The model under review builds one solid part; all positions refer to its coordinate system, in mm. Face numbers are marked on the shaded views. Give positions to 0.01 mm unless a question says otherwise; leave off trailing zeros. Write each loop counter-clockwise with the first axis right and the second up, starting at its lowest first coordinate (ties: lowest second). Pieces come first, ordered by that corner, then holes. Notation, with made-up numbers: (48.25, 59) - (91.25, 59) arc R30 cw to (91.25, 88) - close; hole circle Ø6 at (34, -25.75). An arc over 180 degrees is marked (long way). One line per question, with ' | ' between items. Start each with the question number.
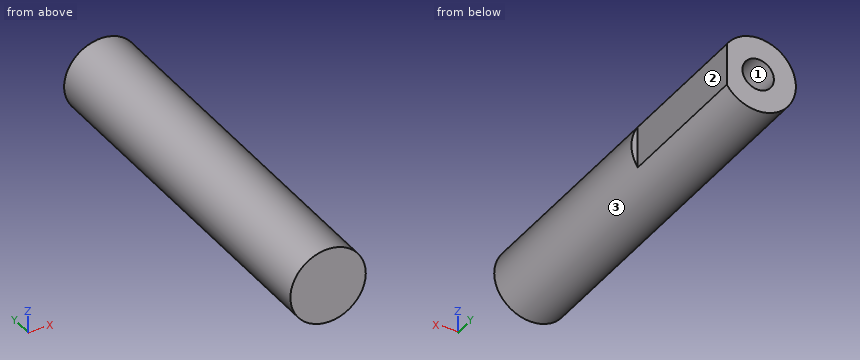
```python
from build123d import *

# Parameters (mm, degrees)
SKETCH1_R                 = 3
SHAFT_DEPTH               = 20.5
SHAFT_DEPTH_BACK          = 10
SKETCH2_W                 = 0.5
SKETCH2_H                 = 6
KEY_DEPTH                 = 12
M3X0_5_TAPPED_HOLE1_D     = 2.5
M3X0_5_TAPPED_HOLE1_DEPTH = 14.5
M3X0_5_TAPPED_HOLE1_TIP   = 0.751075774


with BuildPart() as part:
    # Sketch1 → SHAFT (new body, two sides)
    with BuildSketch(Plane(origin=(0, 0, 0), x_dir=(1, 0, 0), z_dir=(0, 1, 0))) as shaft_sk:
        Circle(SKETCH1_R)
    extrude(amount=SHAFT_DEPTH)
    extrude(shaft_sk.sketch, amount=-SHAFT_DEPTH_BACK)

    # Sketch2 → KEY (cut)
    with BuildSketch(Plane(origin=(0, 20.5, 0), x_dir=(1, 0, 0), z_dir=(0, 1, 0))):
        with Locations((2.75, 0)):
            Rectangle(SKETCH2_W, SKETCH2_H)
    extrude(amount=-KEY_DEPTH, mode=Mode.SUBTRACT)

    # M3x0.5 Tapped Hole1
    with Locations(Plane(origin=(0, 20.5, 0), x_dir=(1, 0, 0), z_dir=(0, 1, 0))):
        with Locations((0, 0)):
            Hole(M3X0_5_TAPPED_HOLE1_D / 2, depth=M3X0_5_TAPPED_HOLE1_DEPTH)
            with Locations((0, 0, -(M3X0_5_TAPPED_HOLE1_DEPTH + M3X0_5_TAPPED_HOLE1_TIP / 2))):  # 118° drill point
                Cone(0, M3X0_5_TAPPED_HOLE1_D / 2, M3X0_5_TAPPED_HOLE1_TIP, mode=Mode.SUBTRACT)


solid = part.part
```
Item 1: For probe 1 along Z at (x, y) = (0, 10.75); probe 2 along Z at (x, y) = (0.75, 12.5); probe 3 along Z at (x, y) = (-0.15, -4.5), list the stretches that pass through material, from the lowest coordinate up.
Item 2: Take a section at C-C (z = 2.25). Give the boundary of the cut face in (x, y), plus the area to 3 significant figures.
Item 3: Take a section at D-D (z = -2.3). Give the boundary of the cut face in (x, y), plus the area to 3 significant figures.
Item 4: Take a section at A-A (y = 12). Give the boundary of the cut face in (x, z), plus the area to 3 significant figures.
Item 5: Clearance check with flat-ended pins moving along their axes: P1, Ø2, axis at x = 1.5, y = -1, coming from the -Z side; P2, Ø0.6, axis at x = 3, z = 0.5, coming from the +Y side; P3, Ø1.7, axis at y = 14, z = -1, coming from the +X side. State where each tip first meets the part, or that it passes through.
Item 6: The part is to be moulded in two halves that separate along X. For the marked faces 1, 2 and 3, say which applies: +X half, -X half, draft (parallel to the pull), parting line (faces both ways), or undercut.
Item 7: Take a section at B-B (y = 4). Give the boundary of the cut face in (x, z), plus the area to 3 significant figures.
Check sheet entries:
1) probe 1: z = -3 to -1.25, 1.25 to 3 | probe 2: z = -2.9 to -1, 1 to 2.9 | probe 3: z = -3 to 3
2) outline: (-1.98, -10) - (1.98, -10) - (1.98, 20.5) - (-1.98, 20.5) - close | area: 121 mm^2
3) outline: (-1.93, -10) - (1.93, -10) - (1.93, 20.5) - (-1.93, 20.5) - close | area: 117 mm^2
4) outline: (2.5, -1.66) - (2.5, 1.66) arc R3 ccw (long way) to start; hole circle Ø2.5 at (0, 0) | area: 22.2 mm^2
5) P1: stops at z = -2.96 | P2: stops at y = 8.5 | P3: stops at x = 2.5
6) face 1: undercut | face 2: +X half | face 3: parting line
7) outline: circle Ø6 at (0, 0) | area: 28.3 mm^2
